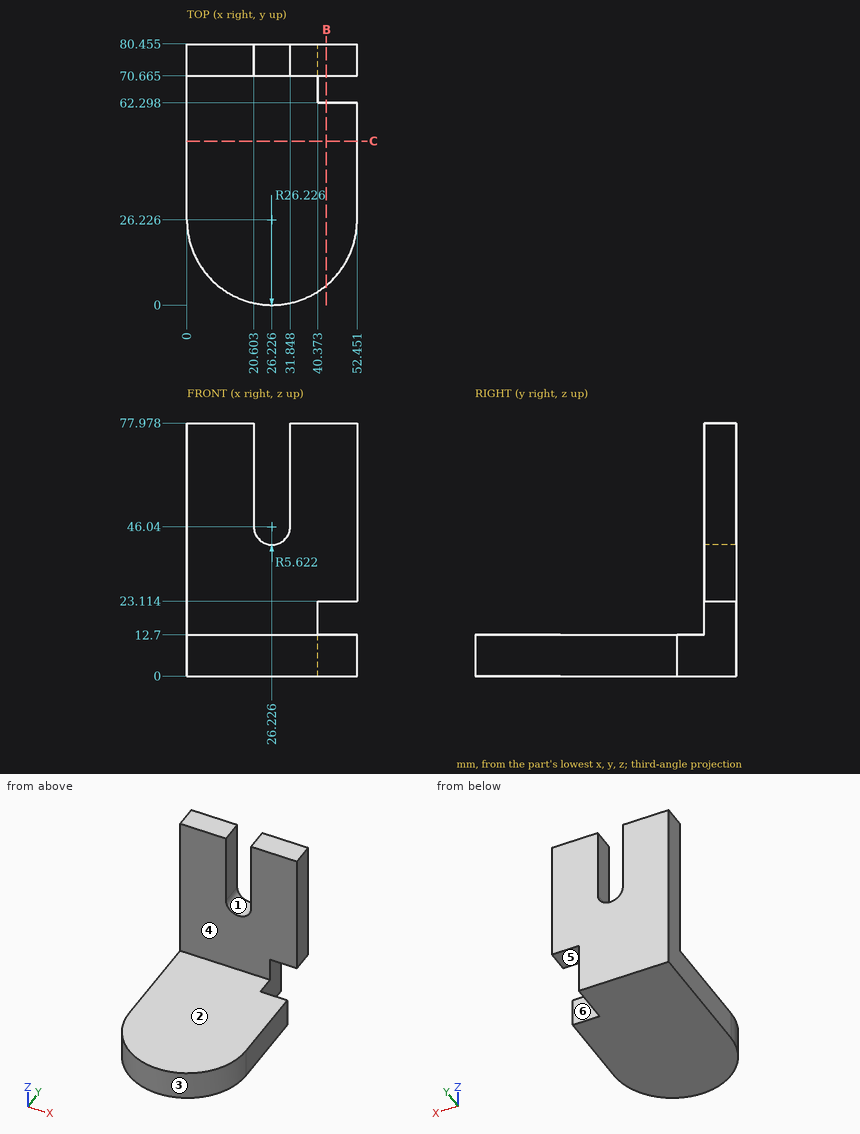
Here's the drawing with two shaded views (mm, measured from the low corner). I have some questions. A direction names the side the tool comes from. Coordinates: 2 decimals unless noted, no trailing zeros. Loops run counter-clockwise (first coordinate to the right, second up) from the corner with the lowest first, then second, coordinate; pieces in that order, holes last. Notation, with made-up numbers: M 31.25,46 L 75.25,46 A21 ccw 75.25,50 Z; hole C 6.5,30 d6. An arc over 180 degrees is marked long. Return JSON: item names as keys, results as strings. Group by question number.
Item 1: Imagine slicing it at B-B (x = 43). Please give me the cut outline in (y, z) (1 decimal), and give its area (3 significant figures).
Item 2: Imagine slicing it at C-C (y = 50.5). Please give me the cut outline in (x, z), and give its area (3 significant figures).
Item 3: I'm going to push flat-ended pins straight in: pin 1 Ø12 at (x, y) = (13, 62) entering from +Z; pin 2 Ø6 at (x, z) = (46.5, 9.5) entering from +Y; pin 3 Ø9 at (y, z) = (73.5, 6.5) entering from +X; pin 4 Ø4 at (x, y) = (43.5, 67) entering from -Z. Where does each tip first touch, or does it pass through?
Item 4: If I drill on L1, parallel to X at y = 73, z = 46.5; L2, parallel to Y at x = 40.5, z = 44.5 (1 decimal); L3, parallel to X at y = 76, z = 11, over which ranges is the centre line in solid material (lowest first)? Write a range as from..to.
Item 5: On a 3-axis mill with a long thin cutter (end or side, diameter ignored), from which of +Z, -Z, +X, -X, +Y, -Y can I reach the whole of each face in a straight line? I mean the marked faces 4, 5 and 6. Say none if no direction works.
Item 6: Thinking about a two-plate mould opening in X: for the marked faces 1, 2 and 3, which applies, released by +X, released by -X, zero draft, split by the parting line, or undercut?
Verdict:
{
 "1": {"outline": "M 6.1,0 L 62.3,0 L 62.3,12.7 L 6.1,12.7 Z; M 70.7,23.1 L 80.5,23.1 L 80.5,78 L 70.7,78 Z", "area": "1,250 mm^2"},
 "2": {"outline": "M 0,0 L 52.45,0 L 52.45,12.7 L 0,12.7 Z", "area": "666 mm^2"},
 "3": {"pin 1": "stops at z = 12.7", "pin 2": "stops at y = 62.3", "pin 3": "stops at x = 40.37", "pin 4": "passes through"},
 "4": {"L1": "x = 0..20.6, 31.85..52.45", "L2": "y = 70.7..80.5", "L3": "x = 0..40.37"},
 "5": {"face 4": "+Z, +X, -X, -Y", "face 5": "-Z, +X, +Y, -Y", "face 6": "+Z, -Z, +X, +Y"},
 "6": {"face 1": "undercut", "face 2": "zero draft", "face 3": "split by the parting line"}
}
